Verification items for this drawing (mm, ordinates from the low corner). A direction names the side the tool comes from. Give positions to 0.01 mm unless a question says otherwise; leave off trailing zeros. Loops run counter-clockwise (first coordinate to the right, second up) from the corner with the lowest first, then second, coordinate; pieces in that order, holes last. Notation, with made-up numbers: M 1.25,51.5 L 53.25,51.5 A23 ccw 53.25,64.5 Z; hole C 75.25,0.5 d1. An arc over 180 degrees is marked long. Use a Markdown table: item, result.
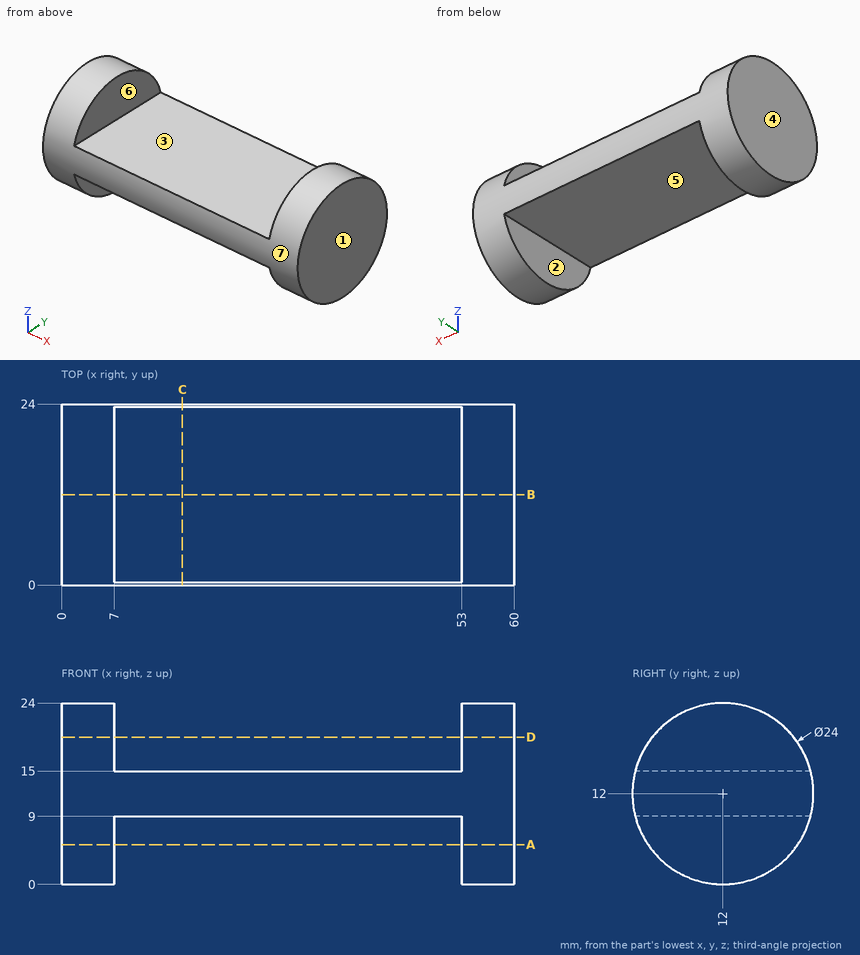
(1) Gauge pin test, flat ends, axial feed: P1, Ø12, axis at x = 29.5, y = 6.5, coming from the -Z side; P2, Ø4, axis at x = 50, z = 7.5, coming from the -Y side; P3, Ø5, axis at x = 38.5, y = 16, coming from the +Z side. Record the tip position at first contact, or that the pin passes through.
Results below:
| item | result |
|---|---|
| P1 | z = 9 |
| P2 | y = 0.26 |
| P3 | z = 15 |
(2) Draft check along X on the marked faces 1, 2, 3 and 4. Enter one of: +X half, -X half, draft (parallel to the pull), parting line (faces both ways), or undercut.
Results below:
| item | result |
|---|---|
| face 1 | +X half |
| face 2 | undercut |
| face 3 | undercut |
| face 4 | -X half |
(3) Material ranges on line 1 (X direction, y = 14.75, z = 8.5); line 2 (Y direction, x = 55.5, z = 11.75); line 3 (Z direction, x = 9, y = 15.75), recorded low to high.
Results below:
| item | result |
|---|---|
| line 1 | 0 to 7, 53 to 60 |
| line 2 | 0 to 24 |
| line 3 | 9 to 15 |
(4) Cross-section at D-D on z = 19.5. Record the cut outline in (x, y).
Results below:
| item | result |
|---|---|
| outline | M 0,2.63 L 7,2.63 L 7,21.37 L 0,21.37 Z; M 53,2.63 L 60,2.63 L 60,21.37 L 53,21.37 Z |
(5) Set-up check for the marked faces 5, 6 and 7: record each of +Z, -Z, +X, -X, +Y, -Y from which the full face is reachable in a straight line by a thin tool's end or side.
Results below:
| item | result |
|---|---|
| face 5 | -Z, +Y, -Y |
| face 6 | +Z, +Y, -Y |
| face 7 | +X, -X |
(6) Cross-section at B-B on y = 12. Record the cut outline in (x, z).
Results below:
| item | result |
|---|---|
| outline | M 0,0 L 7,0 L 7,9 L 53,9 L 53,0 L 60,0 L 60,24 L 53,24 L 53,15 L 7,15 L 7,24 L 0,24 Z |
(7) Cross-section at A-A on z = 5.25. Record the cut outline in (x, y).
Results below:
| item | result |
|---|---|
| outline | M 0,2.08 L 7,2.08 L 7,21.92 L 0,21.92 Z; M 53,2.08 L 60,2.08 L 60,21.92 L 53,21.92 Z |
(8) Cross-section at C-C on x = 16. Record the cut outline in (y, z).
Results below:
| item | result |
|---|---|
| outline | M 0.38,9 L 23.62,9 A12 ccw 23.62,15 L 0.38,15 A12 ccw Z |
